Geometry check sheet. Reference: the model listing, model coordinates, mm. Face numbers are marked on the shaded views. A direction names the side the tool comes from. Coordinates: 2 decimals unless noted, no trailing zeros. Write each loop counter-clockwise with the first axis right and the second up, starting at its lowest first coordinate (ties: lowest second). Pieces come first, ordered by that corner, then holes. Notation, with made-up numbers: M -7.5,-22.5 L 10.5,-22.5 A36 ccw 10.5,15.5 Z; hole C 83,15.25 d1. An arc over 180 degrees is marked long. Answer as a JSON object with one key per item and string values. Group by question number.
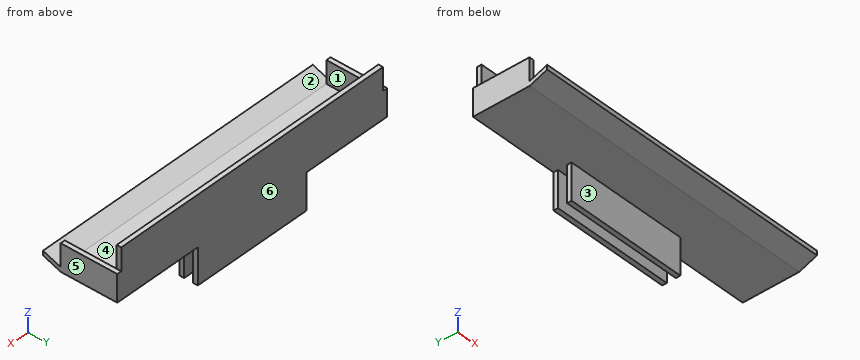
```python
from build123d import *

# Parameters (mm, degrees)
CROQUIS1_W              = 65
CROQUIS1_H              = 10.5
SALIENTE_EXTRUIR1_DEPTH = 1
CROQUIS5_W              = 67
CROQUIS5_H              = 12.5
CROQUIS5_W_2            = 65
CROQUIS5_H_2            = 10.5
SALIENTE_EXTRUIR3_DEPTH = 6
CROQUIS6_W              = 27
CROQUIS6_H              = 1
SALIENTE_EXTRUIR4_DEPTH = 8
CROQUIS7_W              = 65
CROQUIS7_H              = 1
CORTAR_EXTRUIR1_DEPTH   = 5
SALIENTE_EXTRUIR5_DEPTH = 67
CROQUIS9_W              = 65
CROQUIS9_H              = 1
SALIENTE_EXTRUIR6_DEPTH = 5


with BuildPart() as part:
    # Croquis1 → Saliente-Extruir1 (new body)
    with BuildSketch(Plane.XY):
        with Locations((-41.330573237, 12.632352941)):
            Rectangle(CROQUIS1_W, CROQUIS1_H)
    extrude(amount=SALIENTE_EXTRUIR1_DEPTH)

    # Croquis5 → Saliente-Extruir3 (add)
    with BuildSketch(Plane(origin=(0, 0, 0), x_dir=(-1, 0, 0), z_dir=(0, 0, -1))):
        with Locations((41.330573237, 12.632352941)):
            Rectangle(CROQUIS5_W, CROQUIS5_H)
        with Locations((41.330573237, 12.632352941)):
            Rectangle(CROQUIS5_W_2, CROQUIS5_H_2, mode=Mode.SUBTRACT)
    extrude(amount=-SALIENTE_EXTRUIR3_DEPTH)

    # Croquis6 → Saliente-Extruir4 (add)
    with BuildSketch(Plane(origin=(0, 0, 0), x_dir=(-1, 0, 0), z_dir=(0, 0, -1))):
        with Locations((41.330573237, 18.382352941)):
            Rectangle(CROQUIS6_W, CROQUIS6_H)
        with Locations((41.330573237, 15.382352941)):
            Rectangle(CROQUIS6_W, CROQUIS6_H)
    extrude(amount=SALIENTE_EXTRUIR4_DEPTH)

    # Croquis7 → Cortar-Extruir1 (cut)
    with BuildSketch(Plane.XY.offset(6)):
        with Locations((-41.330573237, 6.882352941)):
            Rectangle(CROQUIS7_W, CROQUIS7_H)
    extrude(amount=-CORTAR_EXTRUIR1_DEPTH, mode=Mode.SUBTRACT)

    # Croquis8 → Saliente-Extruir5 (add)
    with BuildSketch(Plane(origin=(-7.830573237, 0, 0), x_dir=(0, 0, -1), z_dir=(1, 0, 0))):
        Polygon((0, 6.382352941), (-1.000715145, 6.382352941), (-2.414928707, 2.468139379), (-1.414213562, 2.468139379), align=None)
    extrude(amount=-SALIENTE_EXTRUIR5_DEPTH)

    # Croquis9 → Saliente-Extruir6 (add)
    with BuildSketch(Plane.XY.offset(6)):
        with Locations((-41.330573237, 18.382352941)):
            Rectangle(CROQUIS9_W, CROQUIS9_H)
    extrude(amount=SALIENTE_EXTRUIR6_DEPTH)


solid = part.part
```
1) Section check C-C (y = 12). Record the cut outline in (x, z), then the cut area to 3 significant figures.
2) Material ranges on probe 1 along Y at (x, z) = (-49.5, -2.5); probe 2 along X at (y, z) = (12.25, 4); probe 3 along Y at (x, z) = (-56, 9), recorded low to high. Write a range as [from, to].
3) Go/stop test with flat-tipped pins: pin 1 Ø0.5 at (y, z) = (18.5, 9.5) entering from +X; pin 2 Ø1.1 at (x, y) = (-8.5, 10.5) entering from +Z; pin 3 Ø8 at (x, y) = (-38.5, 7.5) entering from +Z; pin 4 Ø1 at (y, z) = (12.5, -4.5) entering from +X. Record where each tip stops, or that it passes through.
4) Set-up check for the marked faces 1, 2 and 3: record each of +Z, -Z, +X, -X, +Y, -Y from which the full face is reachable in a straight line by a thin tool's end or side.
5) Section check A-A (z = -3). Record the cut outline in (x, y).
6) Draft check along Y on the marked faces 4, 5 and 6. Enter one of: +Y half, -Y half, draft (parallel to the pull), parting line (faces both ways), or undercut.
Entries:
{
 "1": {"outline": "M -74.83,0 L -7.83,0 L -7.83,6 L -8.83,6 L -8.83,1 L -73.83,1 L -73.83,6 L -74.83,6 Z", "area": "77.0 mm^2"},
 "2": {"probe 1": "[14.88, 15.88], [17.88, 18.88]", "probe 2": "[-74.83, -73.83], [-8.83, -7.83]", "probe 3": "[17.88, 18.88]"},
 "3": {"pin 1": "x = -8.83", "pin 2": "z = 6", "pin 3": "z = 2.04", "pin 4": "through"},
 "4": {"face 1": "+Z", "face 2": "+Z, +X, -X", "face 3": "-Z, +X, -X, -Y"},
 "5": {"outline": "M -54.83,14.88 L -27.83,14.88 L -27.83,15.88 L -54.83,15.88 Z; M -54.83,17.88 L -27.83,17.88 L -27.83,18.88 L -54.83,18.88 Z"},
 "6": {"face 4": "undercut", "face 5": "draft", "face 6": "+Y half"}
}
